Check sheet for the modelled part. Datum: model origin and axes. Units: mm. A direction names the side the tool comes from. Coordinates: 2 decimals unless noted, no trailing zeros. Loops run counter-clockwise (first coordinate to the right, second up) from the corner with the lowest first, then second, coordinate; pieces in that order, holes last.
Autodesk Fusion 360 part; units mm, degrees
sketch "Sketch1" plane through (0, 0, 0) normal (0, 0, 1) x (1, 0, 0)
  line L0 (0, 0) -> (-98, 0)
  line L1 (-98, 0) -> (-98, -42)
  line L2 (-98, -42) -> (0, -42)
  line L3 (0, -42) -> (0, 0)
  line L4 (0, 0) -> (-14, 0)
  line L5 (0, 0) -> (-14, 0)
  line L6 (-14, 0) -> (-14, -42)
  line L7 (-14, -42) -> (0, -42)
  line L8 (0, -42) -> (0, 0)
  line L9 (-98, 0) -> (-84, 0)
  line L10 (-98, 0) -> (-98, -42)
  line L11 (-84, 0) -> (-98, 0)
  line L12 (-98, 0) -> (-98, -42)
  line L13 (-98, -42) -> (-84, -42)
  line L14 (-84, -42) -> (-84, 0)
  dimension "d1" = 98
  dimension "d2" = 42
  dimension "d3" = 14
  dimension "d4" = 14
  dimension "d5" = 14
extrude "Extrude1" add sketch "Sketch1" along normal blind 20
extrude "Extrude2" cut sketch "Sketch1" along normal blind 9 contours L0 L2 L6 L14
sketch "Sketch2" plane through (0, 0, 0) normal (0, 0, 1) x (1, 0, 0)
sketch "Sketch3" plane through (0, 0, 20) normal (0, 0, 1) x (-1, 0, 0)
  line L0 (98, 42) -> (0, 42)
  line L1 (0, 42) -> (0, 0)
  line L2 (0, 0) -> (98, 0)
  line L3 (98, 0) -> (98, 42)
  line L4 (0, 0) -> (24, 0)
  line L5 (24, 0) -> (24, 42)
  line L6 (24, 42) -> (0, 42)
  line L7 (0, 42) -> (0, 0)
  circle A0 centre (24, 21) radius 6
  line L8 (98, 0) -> (74, 0)
  line L9 (74, 0) -> (74, 42)
  line L10 (74, 42) -> (98, 42)
  line L11 (98, 42) -> (98, 0)
  circle A1 centre (74, 21) radius 6
  dimension "d10" = 24
  dimension "d11" = 42
  dimension "d12" = 12
  dimension "d13" = 24
  dimension "d14" = 12
extrude "Extrude3" cut sketch "Sketch3" against normal blind 15 contours L5 A0 | L5 A0
extrude "Extrude4" cut sketch "Sketch3" against normal blind 15 contours L9 A1 | L9 A1
sketch "Sketch4" plane through (0, 0, 20) normal (0, 0, 1) x (-1, 0, 0)
  line L0 (74, 0) -> (24, 0)
  line L1 (24, 0) -> (24, 42)
  line L2 (24, 42) -> (74, 42)
  line L3 (74, 42) -> (74, 0)
extrude "Extrude5" add sketch "Sketch3" along normal blind 40 contours L0 L2 L5 A0 L9 A1
sketch "Sketch5" plane through (0, 0, 60) normal (0, 0, 1) x (-1, 0, 0)
  line L0 (24, 0) -> (74, 0)
  line L1 (74, 0) -> (74, 15)
  arc A0 (74, 27) -> (74, 15) centre (74, 21) ccw
  line L2 (74, 27) -> (74, 42)
  line L3 (74, 42) -> (24, 42)
  line L4 (24, 42) -> (24, 27)
  arc A1 (24, 15) -> (24, 27) centre (24, 21) ccw
  line L5 (24, 15) -> (24, 0)
  line L6 (74, 0) -> (24, 0)
  line L7 (24, 0) -> (24, 42)
  line L8 (24, 42) -> (74, 42)
  line L9 (74, 42) -> (74, 0)
  line L10 (74, 0) -> (49, 0)
  line L11 (74, 0) -> (49, 0)
  line L12 (49, 0) -> (49, 42)
  line L13 (49, 42) -> (74, 42)
  line L14 (74, 42) -> (74, 0)
  line L15 (49, 0) -> (42, 0)
  line L16 (42, 0) -> (42, 42)
  line L17 (42, 42) -> (49, 42)
  line L18 (49, 42) -> (49, 0)
  line L19 (49, 0) -> (56, 0)
  line L20 (56, 0) -> (56, 42)
  line L21 (56, 42) -> (49, 42)
  line L22 (49, 42) -> (49, 0)
  dimension "d21" = 25
  dimension "d22" = 7
  dimension "d23" = 7
extrude "Extrude6" cut sketch "Sketch5" against normal blind 40 contours L0 L1 A0 L2 L3 L6 L8 L9 L10 L11 L13 L14 L20
extrude "Extrude7" cut sketch "Sketch5" against normal blind 40 contours L0 L3 L4 A1 L5 L6 L7 L8 L16
sketch "Sketch6" plane through (0, 0, 60) normal (0, 0, 1) x (-1, 0, 0)
fillet "Fillet1" radius 5 1 edges at (-98, -21, 20)
fillet "Fillet2" radius 5 1 edges at (0, -21, 20)
fillet "Fillet3" radius 21 1 edges at (-49, 0, 60)
fillet "Fillet4" radius 21 1 edges at (-49, -42, 60)
sketch "Sketch7" plane through (-42, 0, 0) normal (1, 0, 0) x (0, 1, 0)
  arc A0 (0, 39) -> (-42, 39) centre (-21, 39) ccw
  line L0 (-42, 39) -> (-42, 20)
  line L1 (-42, 20) -> (0, 20)
  line L2 (0, 20) -> (0, 39)
  line L3 (-42, 39) -> (0, 39)
  line L4 (0, 39) -> (0, 20)
  line L5 (0, 20) -> (-42, 20)
  line L6 (-42, 20) -> (-42, 39)
  circle A1 centre (-21, 39) radius 10
  dimension "d36" = 20
extrude "Extrude8" cut sketch "Sketch7" against normal blind 14 contours L3 A1 | L3 A1
(1) Section check C-C, the plane z = 17. Enter the section's corners in (x, y).
(2) Scan lines: line 1 along X through (y, z) = (-21, 15); line 2 along X through (y, z) = (-35, 2.5); line 3 along Y through (x, z) = (-24, 13.25). Record each from-to range of solid material in increasing order.
(3) Gauge pin test, flat ends, axial feed: P1, Ø10, axis at y = -11.5, z = 22, coming from the +X side; P2, Ø1.5, axis at x = -51.5, z = 48, coming from the -Y side; P3, Ø6, axis at y = -5.5, z = 51, coming from the +X side; P4, Ø6, axis at x = -15.5, z = 15.5, coming from the +Y side. Record the tip position at first contact, or that the pin passes through.
(4) Section check B-B, the plane z = 38. Enter the section's corners in (x, y), plus the area to 3 significant figures.
(5) Section check A-A, the plane x = -74. Enter the section's corners in (y, z), plus the area to 3 significant figures.
(6) Draft check along X on faces 6 (the face through (-68, -21, 15)), 7 (the face through (-79, -16, 20)), 8 (the face through (-96, -21, 19)), 9 (the face through (-42, -11, 36)). Enter one of: pulls with the +X half, pulls with the -X half, needs draft (parallel to the pull), parting line crosses it, or undercut.
(7) Section check D-D, the plane y = -6. Enter the section's corners in (x, z), plus the area to 3 significant figures.
(8) Set-up check for faces 1 (the face through (-19.24, -17.35, 14.58)), 2 (the face through (-48.902, -16.386, 30.128)), 3 (the face through (-14, -21, 4)), 4 (the face through (-56, -11, 36)), 5 (the face through (-20, -16, 20)): record each of +Z, -Z, +X, -X, +Y, -Y from which the full face is reachable in a straight line by a thin tool's end or side.
Determined:
1. outline: (-97.58, -42) - (-0.42, -42) - (-0.42, 0) - (-97.58, 0) - close; hole circle Ø12 at (-74, -21); hole circle Ø12 at (-24, -21)
2. line 1: x = -98 to -80, -68 to -30, -18 to 0
2. line 2: x = -98 to -84, -14 to 0
2. line 3: y = -42 to -27, -15 to 0
3. P1: stops at x = -0.42
3. P2: stops at y = -40.31
3. P3: stops at x = -42
3. P4: stops at y = 0
4. outline: (-56, -42) - (-42, -42) - (-42, -30.95) - (-56, -30.95) - close; (-56, -11.05) - (-42, -11.05) - (-42, 0) - (-56, 0) - close
4. area: 309 mm2
5. outline: (-42, 9) - (-27, 9) - (-27, 20) - (-42, 20) - close; (-15, 9) - (0, 9) - (0, 20) - (-15, 20) - close
5. area: 330 mm2
6. face 6: undercut
6. face 7: needs draft
6. face 8: pulls with the -X half
6. face 9: pulls with the +X half
7. outline: (-98, 0) - (-84, 0) - (-84, 9) - (-14, 9) - (-14, 0) - (0, 0) - (0, 15) arc R5 ccw to (-5, 20) - (-42, 20) - (-42, 53.7) - (-56, 53.7) - (-56, 20) - (-93, 20) arc R5 ccw to (-98, 15) - close
7. area: 1,790 mm2
8. face 1: +Z, -Z
8. face 2: +X, -X
8. face 3: -Z, +Y, -Y
8. face 4: +Z, -X, +Y, -Y
8. face 5: +Z, +X, +Y, -Y
